```python
from build123d import *

# Parameters (mm, degrees)
EXTRUDE1_REACH             = 26.46
SKETCH2_W                  = 2
SKETCH2_H                  = 2
EXTRUDE1_DIRECTION_2_REACH = 26.46


with BuildPart() as part:
    # Sketch1 → Revolve1 (revolve)
    with BuildSketch(Plane.XY, mode=Mode.PRIVATE) as revolve1_sk:
        Polygon((-3, 0), (-3, 18), (-5.886751346, 23), (0, 23), (0, 0), (0, -1.732050808), align=None)
    revolve(revolve1_sk.sketch.rotate(Axis((0, 0, 0), (0, 1, 0)), 270), axis=Axis((0, 0, 0), (0, 1, 0)))

    # Extrude1: up to this cone (the profile starts inside it)
    extrude1_end = Plane(origin=(0, 22, 0), z_dir=(0, 1, 0)).offset(-9.196151423) * Cone(1e-06, 23.940148475, 41.465552499, align=(Align.CENTER, Align.CENTER, Align.MIN), mode=Mode.PRIVATE)
    # Sketch2 → Extrude1 (cut, up to the surface)
    with BuildSketch(Plane.XY, mode=Mode.PRIVATE) as extrude1_sk1:
        with Locations((0, 22)):
            Rectangle(SKETCH2_W, SKETCH2_H)
    extrude1_tool1 = extrude(extrude1_sk1.sketch, amount=-EXTRUDE1_REACH, mode=Mode.PRIVATE) & extrude1_end
    add(extrude1_tool1.solids().sort_by_distance((0, 22, 0))[0], mode=Mode.SUBTRACT)

    # Extrude1 direction 2: up to this cone (the profile starts inside it)
    extrude1_direction_2_end = Plane(origin=(0, 22, 0), z_dir=(0, 1, 0)).offset(-9.196151423) * Cone(1e-06, 23.940148475, 41.465552499, align=(Align.CENTER, Align.CENTER, Align.MIN), mode=Mode.PRIVATE)
    # Sketch2 → Extrude1 direction 2 (cut, up to the surface)
    with BuildSketch(Plane.XY, mode=Mode.PRIVATE) as extrude1_direction_2_sk1:
        with Locations((0, 22)):
            Rectangle(SKETCH2_W, SKETCH2_H)
    extrude1_direction_2_tool1 = extrude(extrude1_direction_2_sk1.sketch, amount=EXTRUDE1_DIRECTION_2_REACH, mode=Mode.PRIVATE) & extrude1_direction_2_end
    add(extrude1_direction_2_tool1.solids().sort_by_distance((0, 22, 0))[0], mode=Mode.SUBTRACT)


solid = part.part
```
Can you work these out from the model? Positions are in its coordinate system, mm. A direction names the side the tool comes from. Coordinates: 2 decimals unless noted, no trailing zeros. Write each loop counter-clockwise with the first axis right and the second up, starting at its lowest first coordinate (ties: lowest second). Pieces come first, ordered by that corner, then holes. Notation, with made-up numbers: (58, 88) - (87, 88) arc R23 cw to (87, 116) - close; hole circle Ø8 at (-34.75, 48.25). An arc over 180 degrees is marked (long way). Return JSON: item names as keys, results as strings.
Q1. I'm going to push flat-ended pins straight in: pin 1 Ø2 at (y, z) = (6, 3) entering from +X; pin 2 Ø6 at (x, y) = (2, 19) entering from -Z; pin 3 Ø0.6 at (y, z) = (22, 0.5) entering from -X. Where does each tip first touch, or does it pass through?
Computed values:
{"pin 1": "stops at x = 2.24", "pin 2": "stops at z = -5.11", "pin 3": "stops at x = -5.46"}
Q2. Please list where these lines run through material, in increasing order: L1, parallel to X at y = 21.25, z = 3.5; L2, parallel to X at y = 10.5, z = -1.5; L3, parallel to Y at x = -3.75, z = 0.5. Write a range as from..to.
Computed values:
{"L1": "x = -3.4..-1, 1..3.4", "L2": "x = -2.6..2.6", "L3": "y = 19.36..23"}
Q3. If we section it at B-B (y = 20.25): Please give me the cut outline in (x, z).
Computed values:
{"outline": "circle Ø8.6 at (0, 0)"}
Q4. Thinking about a two-plate mould opening in X: for faces 1 (the flat face through (-3, 23, 0)), 2 (the flat face through (-1, 22, 0)), 3 (the cylindrical face through (-0.9, 9.13, -2.86)), 4 (the flat face through (0, 21, 0)), which applies, +X half, -X half, draft (parallel to the pull), parting line (faces both ways), or undercut?
Computed values:
{"face 1": "draft", "face 2": "undercut", "face 3": "parting line", "face 4": "undercut"}
Q5. If we section it at A-A (y = 5): Please give me the cut outline in (x, z).
Computed values:
{"outline": "circle Ø6 at (0, 0)"}
Q6. On a 3-axis mill with a long thin cutter (end or side, diameter ignored), from which of +Z, -Z, +X, -X, +Y, -Y can I reach the whole of each face in a straight line? I mean faces 5 (the conical face through (1.341, 18.868, -3.234)), 6 (the flat face through (1, 22, 0)). Say none if no direction works.
Computed values:
{"face 5": "-Y", "face 6": "+Z, -Z, +Y"}
